from build123d import *

# Parameters (mm, degrees)
BOSS_EXTRUDE1_DEPTH = 12.25
BOSS_EXTRUDE2_DEPTH = 5
LPATTERN1_COUNT     = 2
LPATTERN1_PITCH     = 17.25
FILLET11_R          = 10
FILLET12_R          = 10


with BuildPart() as part:
    # Sketch1 → Boss-Extrude1 (new body)
    with BuildSketch(Plane.XY):
        with BuildLine():
            Line((0, 19.25), (15, 19.25))
            Line((15, 19.25), (15, 14.25))
            Line((15, 14.25), (0, 14.25))
            ThreePointArc((0, 14.25), (-14.25, 0), (0, -14.25))
            Line((0, -14.25), (15, -14.25))
            Line((15, -14.25), (15, -19.25))
            Line((15, -19.25), (0, -19.25))
            ThreePointArc((0, -19.25), (-19.25, 0), (0, 19.25))
        make_face()
    extrude(amount=BOSS_EXTRUDE1_DEPTH)

    # Sketch2 → Boss-Extrude2 (add)
    with BuildSketch(Plane.XY.offset(12.25)):
        with BuildLine():
            Line((0, 19.25), (15, 19.25))
            Line((15, 19.25), (15, 14.25))
            Line((15, 14.25), (15, -14.25))
            Line((15, -14.25), (15, -19.25))
            Line((15, -19.25), (0, -19.25))
            ThreePointArc((0, -19.25), (-19.25, 0), (0, 19.25))
        make_face()
    boss_extrude2 = extrude(amount=BOSS_EXTRUDE2_DEPTH)

    # LPattern1: Boss-Extrude2 ×2
    with Locations(*[(0, 0, -i * LPATTERN1_PITCH) for i in range(1, LPATTERN1_COUNT)]):
        add(boss_extrude2)

    # Fillet11
    fillet11_edges = [part.edges().sort_by_distance(p)[0] for p in [
        (-19.25, 0, 17.25),
        (7.5, -19.25, 17.25),
        (7.5, 19.25, 17.25),
        (-19.25, 0, -5),
        (7.5, -19.25, -5),
        (7.5, 19.25, -5),
    ]]
    fillet(fillet11_edges, radius=FILLET11_R)

    # Fillet12
    # the kernel refuses this fillet: 10 mm, written as the material it takes off along each edge
    with BuildSketch(Plane(origin=(15, -9.25, 7.25), x_dir=(0, -1, 0), z_dir=(0, 0, -1))) as fillet12_piece_1:
        with BuildLine():
            CenterArc((10 - FILLET12_R, FILLET12_R), FILLET12_R, 270, 90)
            Line((10, FILLET12_R), (10, 0))
            Line((10, 0), (10 - FILLET12_R, 0))
        make_face()
    revolve(axis=Axis((15, -9.25, 7.25), (-1, 0, 0)), revolution_arc=90, mode=Mode.SUBTRACT)
    with BuildSketch(Plane(origin=(15, 9.25, 17.25), x_dir=(0, 0, -1), z_dir=(0, -1, 0)), Plane(origin=(15, -9.25, -5), x_dir=(0, 0, 1), z_dir=(0, 1, 0))) as fillet12_piece_2:
        with BuildLine():
            CenterArc((FILLET12_R, -FILLET12_R), FILLET12_R, 90, 90)
            Line((0, -FILLET12_R), (0, 0))
            Line((0, 0), (FILLET12_R, 0))
        make_face()
    extrude(amount=18.5, mode=Mode.SUBTRACT)
    with BuildSketch(Plane(origin=(15, 9.25, 7.25), x_dir=(0, 1, 0), z_dir=(0, 0, -1))) as fillet12_piece_3:
        with BuildLine():
            CenterArc((10 - FILLET12_R, -FILLET12_R), FILLET12_R, 360, 90)
            Line((10, -FILLET12_R), (10, 0))
            Line((10, 0), (10 - FILLET12_R, 0))
        make_face()
    revolve(axis=Axis((15, 9.25, 7.25), (1, 0, 0)), revolution_arc=90, mode=Mode.SUBTRACT)
    with BuildSketch(Plane(origin=(15, 19.25, 7.25), x_dir=(-1, 0, 0), z_dir=(0, 0, -1)), Plane(origin=(15, -19.25, 7.25), x_dir=(0, 1, 0), z_dir=(0, 0, -1))) as fillet12_piece_4:
        with BuildLine():
            CenterArc((FILLET12_R, -FILLET12_R), FILLET12_R, 90, 90)
            Line((0, -FILLET12_R), (0, 0))
            Line((0, 0), (FILLET12_R, 0))
        make_face()
    extrude(amount=2.25, mode=Mode.SUBTRACT)
    with BuildSketch(Plane(origin=(15, 9.25, 5), x_dir=(0, 1, 0), z_dir=(0, 0, 1))) as fillet12_piece_5:
        with BuildLine():
            CenterArc((10 - FILLET12_R, FILLET12_R), FILLET12_R, 270, 90)
            Line((10, FILLET12_R), (10, 0))
            Line((10, 0), (10 - FILLET12_R, 0))
        make_face()
    revolve(axis=Axis((15, 9.25, 5), (-1, 0, 0)), revolution_arc=90, mode=Mode.SUBTRACT)
    with BuildSketch(Plane(origin=(15, -9.25, 5), x_dir=(0, -1, 0), z_dir=(0, 0, 1))) as fillet12_piece_6:
        with BuildLine():
            CenterArc((10 - FILLET12_R, -FILLET12_R), FILLET12_R, 360, 90)
            Line((10, -FILLET12_R), (10, 0))
            Line((10, 0), (10 - FILLET12_R, 0))
        make_face()
    revolve(axis=Axis((15, -9.25, 5), (1, 0, 0)), revolution_arc=90, mode=Mode.SUBTRACT)


solid = part.part
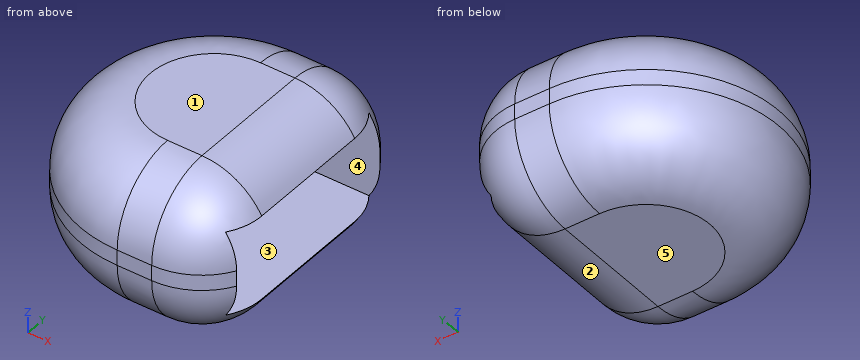
CAD build for the part. Positions are in the model's coordinates, mm. Face numbers are marked on the shaded views. A direction names the side the tool comes from. Round coordinates to 2 decimals unless told otherwise and drop trailing zeros. Write each loop counter-clockwise with the first axis right and the second up, starting at its lowest first coordinate (ties: lowest second). Pieces come first, ordered by that corner, then holes. Notation, with made-up numbers: (43, 26.25) -> (98, 26.25) arc R11 cw to (98, 47.25) -> close; hole circle Ø2 at (46, 33). An arc over 180 degrees is marked (long way). Answer as a JSON object with one key per item and string values.
(1) Pin check, flat tips, straight feed: P1, Ø10, axis at x = 10.5, y = 4.5, coming from the +Z side; P2, Ø6, axis at x = -14.5, y = -1, coming from the -Z side; P3, Ø1, axis at x = -8.5, z = 1.5, coming from the +Y side. Stop position of each tip, or through.
Reported:
{"P1": "stops at z = 17.24", "P2": "stops at z = -4.74", "P3": "stops at y = 16.88"}
(2) Which spindle directions (+Z, -Z, +X, -X, +Y, -Y) get a long thin tool onto all of the face, cutting with end or side? Do the marked faces 4 and 5. Say none if no direction does.
Reported:
{"face 4": "+X", "face 5": "-Z, +X, -X, +Y, -Y"}
(3) Two-plate mould, pull along Z, no slides. Class the marked faces 1, 2 and 3: +Z half, -Z half, draft (parallel to the pull), parting line (faces both ways), or undercut.
Reported:
{"face 1": "+Z half", "face 2": "-Z half", "face 3": "undercut"}
(4) Band-saw the part on A-A, the plane z = 6.75. List the corners of the cut face in (x, y).
Reported:
{"outline": "(0, -19.25) -> (5, -19.25) arc R10 ccw to (13.66, -14.25) -> (0, -14.25) arc R14.25 cw to (0, 14.25) -> (13.66, 14.25) arc R10 ccw to (5, 19.25) -> (0, 19.25) arc R19.25 ccw to start"}
(5) Probe probe 1 along Z at (x, y) = (-5, 5.5); probe 2 along Y at (x, z) = (1.5, 5.25); probe 3 along Y at (x, z) = (-4.5, 9.25). List the from-to ranges inside material, lowest first. Write a range as [from, to].
Reported:
{"probe 1": "z = [-5, 0], [12.25, 17.25]", "probe 2": "y = [-19.25, -14.25], [14.25, 19.25]", "probe 3": "y = [-18.51, -13.52], [13.52, 18.51]"}
